Geometry check sheet. Reference: the model listing, model coordinates, mm. Face numbers are marked on the shaded views. A direction names the side the tool comes from. Round coordinates to 2 decimals unless told otherwise and drop trailing zeros. Order: outer loops, then holes, each group sorted by start corner. A loop starts at its lowest first (then second) coordinate and runs counter-clockwise, first axis right, second up. Notation, with made-up numbers: (79.25, -21.75) -> (105.25, -21.75) arc R23 cw to (105.25, -10.75) -> close; hole circle Ø9 at (18.5, 61). An arc over 180 degrees is marked (long way). Use a Markdown table: item, result. Add a question column.
Item 1: Set-up check for the marked faces 1 and 2: record each of +Z, -Z, +X, -X, +Y, -Y from which the full face is reachable in a straight line by a thin tool's end or side.
Item 2: Sectioned sample at B-B, the plane z = 1.25. Record the cut outline in (x, y) (1 decimal).
Item 3: Material ranges on probe 1 along Z at (x, y) = (0, 0.7); probe 2 along Y at (x, z) = (0, -3.25); probe 3 along Z at (x, y) = (-0.5, 7.25) (1 decimal), recorded low to high. Write a range as [from, to].
Item 4: Sectioned sample at D-D, the plane x = 2.25. Record the cut outline in (y, z) (1 decimal).
Item 5: Sectioned sample at A-A, the plane x = 0. Record the cut outline in (y, z) (1 decimal).
Item 6: Mould release check, pull along X, two halves, no side actions. Record for the marked faces 3, 4 and 5: pulls with the +X half, pulls with the -X half, needs draft (parallel to the pull), parting line crosses it, or undercut.
Item 7: Sectioned sample at C-C, the plane y = 6. Record the cut outline in (x, z) (1 decimal), and give its area (3 significant figures).
Item 8: Gauge pin test, flat ends, axial feed: pin 1 Ø1.9 at (x, z) = (0.5, 2) entering from +Y; pin 2 Ø3 at (x, y) = (1, 5.5) entering from +Z (3 decimals). Record the tip position at first contact, or that the pin passes through.
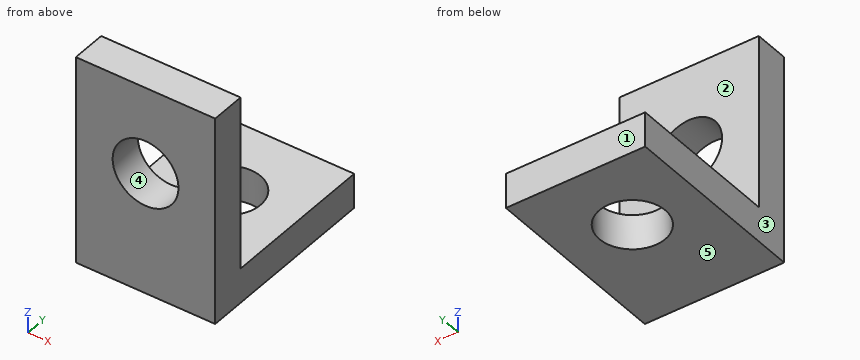
from build123d import *

# Parameters (mm, degrees)
SKETCH1_W                 = 6.35
SKETCH1_H                 = 9.525
BOSS_EXTRUDE1_DEPTH       = 1.5875
SKETCH2_W                 = 6.35
SKETCH2_H                 = 1.5875
BOSS_EXTRUDE2_DEPTH       = 7.1247
F_3_0MM_DOWEL_HOLE1_D     = 3
F_3_0MM_DOWEL_HOLE2_D     = 3
F_3_0MM_DOWEL_HOLE2_DEPTH = 6.35
F_3_0MM_DOWEL_HOLE2_TIP   = 0.901290929


with BuildPart() as part:
    # Sketch1 → Boss-Extrude1 (new body)
    with BuildSketch(Plane(origin=(0, 0, 0), x_dir=(1, 0, 0), z_dir=(0, 1, 0))):
        Rectangle(SKETCH1_W, SKETCH1_H)
    extrude(amount=BOSS_EXTRUDE1_DEPTH)

    # Sketch2 → Boss-Extrude2 (add)
    with BuildSketch(Plane(origin=(0, 1.5875, 0), x_dir=(1, 0, 0), z_dir=(0, 1, 0))):
        with Locations((0, 3.96875)):
            Rectangle(SKETCH2_W, SKETCH2_H)
    extrude(amount=BOSS_EXTRUDE2_DEPTH)

    # Ø3.0mm Dowel Hole1 (through all)
    with Locations(Plane(origin=(0, 1.5875, 0), x_dir=(1, 0, 0), z_dir=(0, 1, 0))):
        with Locations((0, -0.79375)):
            Hole(F_3_0MM_DOWEL_HOLE1_D / 2)

    # Ø3.0mm Dowel Hole2
    with Locations(Plane.XY.offset(-3.175)):
        with Locations((0, 5.14985)):
            Hole(F_3_0MM_DOWEL_HOLE2_D / 2, depth=F_3_0MM_DOWEL_HOLE2_DEPTH)
            with Locations((0, 0, -(F_3_0MM_DOWEL_HOLE2_DEPTH + F_3_0MM_DOWEL_HOLE2_TIP / 2))):  # 118° drill point
                Cone(0, F_3_0MM_DOWEL_HOLE2_D / 2, F_3_0MM_DOWEL_HOLE2_TIP, mode=Mode.SUBTRACT)


solid = part.part
Found:
| question | item | result |
|---|---|---|
| 1 | face 1 | +Z, -Z, +X, -X, +Y |
| 1 | face 2 | +Z, +X, -X, +Y |
| 2 | outline | (-3.2, 0) -> (-1.4, 0) -> (-1.4, 1.6) -> (-3.2, 1.6) -> close; (1.4, 0) -> (3.2, 0) -> (3.2, 1.6) -> (1.4, 1.6) -> close |
| 3 | probe 1 | z = [-4.76, -0.71], [2.29, 4.76] |
| 3 | probe 2 | y = [0, 3.65], [6.65, 8.71] |
| 3 | probe 3 | z = [-4.8, -3.2] |
| 4 | outline | (0, -4.8) -> (8.7, -4.8) -> (8.7, -3.2) -> (1.6, -3.2) -> (1.6, 4.8) -> (0, 4.8) -> close |
| 5 | outline | (0, -4.8) -> (3.6, -4.8) -> (3.6, -3.2) -> (1.6, -3.2) -> (1.6, -0.7) -> (0, -0.7) -> close; (0, 2.3) -> (1.6, 2.3) -> (1.6, 4.8) -> (0, 4.8) -> close; (6.6, -4.8) -> (8.7, -4.8) -> (8.7, -3.2) -> (6.6, -3.2) -> close |
| 6 | face 3 | pulls with the -X half |
| 6 | face 4 | undercut |
| 6 | face 5 | needs draft |
| 7 | outline | (-3.2, -4.8) -> (-1.2, -4.8) -> (-1.2, -3.2) -> (-3.2, -3.2) -> close; (1.2, -4.8) -> (3.2, -4.8) -> (3.2, -3.2) -> (1.2, -3.2) -> close |
| 7 | area | 6.16 mm2 |
| 8 | pin 1 | stops at y = 1.59 |
| 8 | pin 2 | stops at z = -3.175 |
